from build123d import *

# Parameters (mm, degrees)
SKETCH4_W           = 127
SKETCH4_H           = 127
BOSS_EXTRUDE5_DEPTH = 5
SKETCH5_W           = 2
SKETCH5_H           = 1.25
BOSS_EXTRUDE6_DEPTH = 1


with BuildPart() as part:
    # Sketch4 → Boss-Extrude5 (new body)
    with BuildSketch(Plane(origin=(0, 0, 0), x_dir=(1, 0, 0), z_dir=(0, 1, 0))):
        with Locations((-10.766435986, 25.92733564)):
            Rectangle(SKETCH4_W, SKETCH4_H)
    extrude(amount=BOSS_EXTRUDE5_DEPTH)

    # Sketch5 → Boss-Extrude6 (add)
    with BuildSketch(Plane(origin=(0, 5, 0), x_dir=(1, 0, 0), z_dir=(0, 1, 0))):
        with Locations((-41.266435986, -24.94766436)):
            Rectangle(SKETCH5_W, SKETCH5_H)
        with Locations((-61.266435986, -24.94766436)):
            Rectangle(SKETCH5_W, SKETCH5_H)
        with Locations((-21.266435986, -24.94766436)):
            Rectangle(SKETCH5_W, SKETCH5_H)
        with Locations((-1.266435986, -24.94766436)):
            Rectangle(SKETCH5_W, SKETCH5_H)
        with Locations((18.733564014, -24.94766436)):
            Rectangle(SKETCH5_W, SKETCH5_H)
        with Locations((38.733564014, -24.94766436)):
            Rectangle(SKETCH5_W, SKETCH5_H)
        with Locations((-41.266435986, -4.94766436)):
            Rectangle(SKETCH5_W, SKETCH5_H)
        with Locations((-21.266435986, -4.94766436)):
            Rectangle(SKETCH5_W, SKETCH5_H)
        with Locations((-1.266435986, -4.94766436)):
            Rectangle(SKETCH5_W, SKETCH5_H)
        with Locations((18.733564014, -4.94766436)):
            Rectangle(SKETCH5_W, SKETCH5_H)
        with Locations((38.733564014, -4.94766436)):
            Rectangle(SKETCH5_W, SKETCH5_H)
        with Locations((-41.266435986, 15.05233564)):
            Rectangle(SKETCH5_W, SKETCH5_H)
        with Locations((-21.266435986, 15.05233564)):
            Rectangle(SKETCH5_W, SKETCH5_H)
        with Locations((-1.266435986, 15.05233564)):
            Rectangle(SKETCH5_W, SKETCH5_H)
        with Locations((18.733564014, 15.05233564)):
            Rectangle(SKETCH5_W, SKETCH5_H)
        with Locations((38.733564014, 15.05233564)):
            Rectangle(SKETCH5_W, SKETCH5_H)
        with Locations((-41.266435986, 35.05233564)):
            Rectangle(SKETCH5_W, SKETCH5_H)
        with Locations((-21.266435986, 35.05233564)):
            Rectangle(SKETCH5_W, SKETCH5_H)
        with Locations((-1.266435986, 35.05233564)):
            Rectangle(SKETCH5_W, SKETCH5_H)
        with Locations((18.733564014, 35.05233564)):
            Rectangle(SKETCH5_W, SKETCH5_H)
        with Locations((38.733564014, 35.05233564)):
            Rectangle(SKETCH5_W, SKETCH5_H)
        with Locations((-41.266435986, 55.05233564)):
            Rectangle(SKETCH5_W, SKETCH5_H)
        with Locations((-21.266435986, 55.05233564)):
            Rectangle(SKETCH5_W, SKETCH5_H)
        with Locations((-1.266435986, 55.05233564)):
            Rectangle(SKETCH5_W, SKETCH5_H)
        with Locations((18.733564014, 55.05233564)):
            Rectangle(SKETCH5_W, SKETCH5_H)
        with Locations((38.733564014, 55.05233564)):
            Rectangle(SKETCH5_W, SKETCH5_H)
        with Locations((-41.266435986, 75.05233564)):
            Rectangle(SKETCH5_W, SKETCH5_H)
        with Locations((-21.266435986, 75.05233564)):
            Rectangle(SKETCH5_W, SKETCH5_H)
        with Locations((-1.266435986, 75.05233564)):
            Rectangle(SKETCH5_W, SKETCH5_H)
        with Locations((18.733564014, 75.05233564)):
            Rectangle(SKETCH5_W, SKETCH5_H)
        with Locations((38.733564014, 75.05233564)):
            Rectangle(SKETCH5_W, SKETCH5_H)
        with Locations((-61.266435986, -4.94766436)):
            Rectangle(SKETCH5_W, SKETCH5_H)
        with Locations((-61.266435986, 15.05233564)):
            Rectangle(SKETCH5_W, SKETCH5_H)
        with Locations((-61.266435986, 35.05233564)):
            Rectangle(SKETCH5_W, SKETCH5_H)
        with Locations((-61.266435986, 55.05233564)):
            Rectangle(SKETCH5_W, SKETCH5_H)
        with Locations((-61.266435986, 75.05233564)):
            Rectangle(SKETCH5_W, SKETCH5_H)
    extrude(amount=BOSS_EXTRUDE6_DEPTH)


solid = part.part
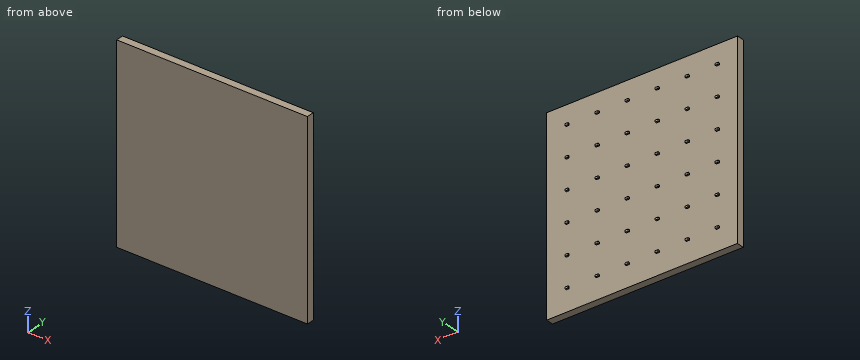
Source: CAD feature listing. Evaluate the final solid. Frame: model axes, mm. Round coordinates to 2 decimals unless told otherwise and drop trailing zeros. Loops run counter-clockwise (first coordinate to the right, second up) from the corner with the lowest first, then second, coordinate; pieces in that order, holes last. Notation, with made-up numbers: (-7, -5.5) -> (21, -5.5) arc R9 cw to (21, -1.5) -> close; hole circle Ø9 at (75, -23). An arc over 180 degrees is marked (long way). Answer as a JSON object with one key per item and string values. Group by question number.
Q1. Contact query for flat-ended pins moving along their axis: P1, Ø1.1, axis at x = 38.5, y = 5.5, coming from the +Z side; P2, Ø0.8, axis at x = 18.5, y = 5.5, coming from the -Z side; P3, Ø0.8, axis at x = 19, y = 5.5, coming from the +Z side; P4, Ø5, axis at x = -52, z = -71, coming from the +Y side. Output: stop coordinate, or through.
Q2. Section query B-B (z = -6). Output: boundary loops of the cut face in (x, y).
Q3. Ray query, line 1 (Y direction, x = -64, z = 30). Return the intervals inside material, ascending. Write a range as from..to.
Q4. Section query A-A (x = 14.5). Output: boundary loops of the cut face in (y, z), plus the area to 3 significant figures.
Completed:
{
 "1": {"P1": "z = 37.57", "P2": "z = -75.68", "P3": "z = 25.57", "P4": "y = 5"},
 "2": {"outline": "(-74.27, 0) -> (52.73, 0) -> (52.73, 5) -> (-74.27, 5) -> close"},
 "3": {"line 1": "0..5"},
 "4": {"outline": "(0, -89.43) -> (5, -89.43) -> (5, 37.57) -> (0, 37.57) -> close", "area": "635 mm²"}
}
